The figure shows three views and two pictorial views of one solid part (mm, origin at its lowest corner). Answer the questions. A direction names the side the tool comes from. Coordinates: 2 decimals unless noted, no trailing zeros. Loops run counter-clockwise (first coordinate to the right, second up) from the corner with the lowest first, then second, coordinate; pieces in that order, holes last. Notation, with made-up numbers: M 55.25,-25.5 L 80.25,-25.5 A12 ccw 80.25,-6.5 Z; hole C -33.75,-34.75 d4. An arc over 180 degrees is marked long. Return JSON: item names as keys, results as strings. Group by question number.
1. Straight lines are drawn through the part: L1, parallel to X at y = 16, z = 12.5; L2, parallel to X at y = 16.75, z = 26.5; L3, parallel to Y at x = 1.5, z = 6. For each, find the intervals that lie inside material, in ascending order. Write a range as from..to.
2. Given P1, Ø8, axis at x = 11.5, z = 13.5, coming from the -Y side; P2, Ø1, axis at x = 1.5, z = 1, coming from the -Y side; P3, Ø0.6, axis at x = 19, y = 1, coming from the -Z side, each flat-ended and moving along its own axis, determine where each tip first touches the part or whether it passes through.
3. Section A-A (y = 17.5) is taken. Write down the section's boundary in (x, z).
4. Section D-D (z = 24.5) is taken. Write down the section's boundary in (x, y).
5. Which of the six approach directions +Z, -Z, +X, -X, +Y, -Y give full straight-line access (tool end or side, diameter ignored) to the marked faces 5, 6, 7 and 8?
6. Section C-C (z = 13) is taken. Write down the section's boundary in (x, y).
7. The mould has two halves that part along X. Classify the marked faces 1, 2, 3 and 4: pulls with the +X half, pulls with the -X half, needs draft (parallel to the pull), parting line crosses it, or undercut.
8. Section B-B (x = 10) is taken. Write down the section's boundary in (y, z).
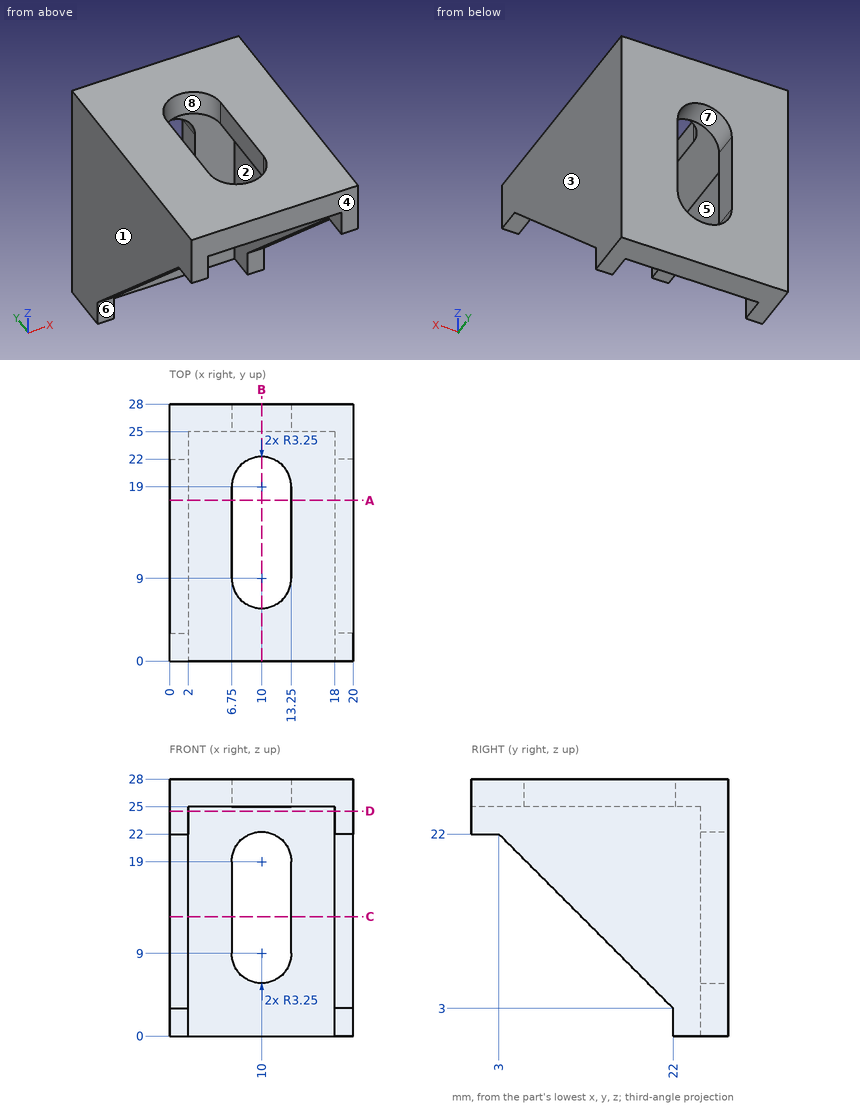
Worked out:
{
 "1": {"L1": "0..2, 18..20", "L2": "0..6.75, 13.25..20", "L3": "19..28"},
 "2": {"P1": "y = 25", "P2": "y = 22", "P3": "z = 22"},
 "3": {"outline": "M 0,7.5 L 2,7.5 L 2,25 L 6.75,25 L 6.75,28 L 0,28 Z; M 13.25,25 L 18,25 L 18,7.5 L 20,7.5 L 20,28 L 13.25,28 Z"},
 "4": {"outline": "M 0,0 L 2,0 L 2,25 L 18,25 L 18,0 L 20,0 L 20,28 L 0,28 Z"},
 "5": {"face 5": "-Z, -Y", "face 6": "-Z, +X, -X, -Y", "face 7": "+Y, -Y", "face 8": "+Z, -Z"},
 "6": {"outline": "M 0,12 L 2,12 L 2,25 L 6.75,25 L 6.75,28 L 0,28 Z; M 13.25,25 L 18,25 L 18,12 L 20,12 L 20,28 L 13.25,28 Z"},
 "7": {"face 1": "pulls with the -X half", "face 2": "undercut", "face 3": "pulls with the +X half", "face 4": "needs draft"},
 "8": {"outline": "M 0,25 L 5.75,25 L 5.75,28 L 0,28 Z; M 22.25,25 L 25,25 L 25,22.25 L 28,22.25 L 28,28 L 22.25,28 Z; M 25,0 L 28,0 L 28,5.75 L 25,5.75 Z"}
}
